The listing builds one solid part. Answer for the finished solid, in the listing's coordinates (mm). Face numbers are marked on the shaded views. A direction names the side the tool comes from. Round coordinates to 2 decimals unless told otherwise and drop trailing zeros. Write each loop counter-clockwise with the first axis right and the second up, starting at its lowest first coordinate (ties: lowest second). Pieces come first, ordered by that corner, then holes.
(1) The mould has two halves that part along X. Classify the marked faces 1, 2 and 3: +X half, -X half, draft (parallel to the pull), parting line (faces both ways), or undercut.
(2) Find the intervals of material crossed by probe 1 along Y at (x, z) = (0, 11); probe 2 along Y at (x, z) = (56.5, -10.5); probe 3 along X at (y, z) = (8, -27), in increasing order.
(3) A cutting plane is placed at A-A, the plane z = -18.5. Give the vertices of the cut face in (x, y).
(4) Each of these flat-tipped pins is pushed along its axis until it touches: pin 1 Ø1.5 at (x, z) = (6, -21.5) entering from -Y; pin 2 Ø8 at (x, z) = (62.5, 24.5) entering from -Y; pin 3 Ø1 at (x, z) = (20.5, 19.5) entering from +Y. Where does it stop, or does it pass through?
(5) A cutting plane is placed at C-C, the plane x = 7. Give the vertices of the cut face in (y, z).
(6) A cutting plane is placed at B-B, the plane y = 0. Give the vertices of the cut face in (x, z), and give its area (4 significant figures).
(7) For the marked faces 4, 5 and 6, determine the directions among +Z, -Z, +X, -X, +Y, -Y from which every point of the face is accessible in a straight line to the end or side of a thin tool.
(8) A cutting plane is placed at D-D, the plane y = 23.5. Give the vertices of the cut face in (x, z).
from build123d import *

# Parameters (mm, degrees)
SKETCH1_R           = 19
BOSS_EXTRUDE1_DEPTH = 32.5
BOSS_EXTRUDE2_START = -9.5
SKETCH2_R           = 5
BOSS_EXTRUDE2_DEPTH = 16
CUT_EXTRUDE2_START  = -16
SKETCH4_R           = 5
CUT_EXTRUDE2_DEPTH  = 16


with BuildPart() as part:
    # Sketch1 → Boss-Extrude1 (new, symmetric)
    with BuildSketch(Plane.XY):
        with BuildLine():
            Line((37.433273968, 19), (50, 19))
            Line((50, 19), (50, 28.5))
            Line((50, 28.5), (0, 28.5))
            ThreePointArc((0, 28.5), (-17.640484356, -22.38444352), (27.710345665, 6.662337662))
            ThreePointArc((27.710345665, 6.662337662), (29.57908326, 15.189643634), (37.433273968, 19))
        make_face()
        Circle(SKETCH1_R, mode=Mode.SUBTRACT)
    extrude(amount=BOSS_EXTRUDE1_DEPTH, both=True)

    # Sketch2 → Boss-Extrude2 (add)
    with BuildSketch(Plane(origin=(0, 28.5, 0), x_dir=(1, 0, 0), z_dir=(0, 1, 0)).offset(BOSS_EXTRUDE2_START)):
        with BuildLine():
            Line((37.5, 20), (37.5, -20))
            ThreePointArc((37.5, -20), (43.725914773, -30.811376164), (56.201736729, -30.853039277))
            Line((56.201736729, -30.853039277), (91.201736729, -10.853039277))
            ThreePointArc((91.201736729, -10.853039277), (97.5, 0), (91.201736729, 10.853039277))
            Line((91.201736729, 10.853039277), (56.201736729, 30.853039277))
            ThreePointArc((56.201736729, 30.853039277), (43.725914773, 30.811376164), (37.5, 20))
        make_face()
        with Locations(Location((50, 20, 0), (0, 0, 270))):
            Circle(SKETCH2_R, mode=Mode.SUBTRACT)
        with Locations(Location((50, -20, 0), (0, 0, 270))):
            Circle(SKETCH2_R, mode=Mode.SUBTRACT)
        with Locations(Location((85, 0, 0), (0, 0, 270))):
            Circle(SKETCH2_R, mode=Mode.SUBTRACT)
    extrude(amount=BOSS_EXTRUDE2_DEPTH)

    # Sketch4 → Cut-Extrude2 (cut)
    with BuildSketch(Plane(origin=(0, 35, 0), x_dir=(1, 0, 0), z_dir=(0, 1, 0)).offset(CUT_EXTRUDE2_START)):
        with Locations(Location((50, -20, 0), (0, 0, 270))):
            Circle(SKETCH4_R)
        with Locations(Location((85, 0, 0), (0, 0, 270))):
            Circle(SKETCH4_R)
        with Locations(Location((50, 20, 0), (0, 0, 270))):
            Circle(SKETCH4_R)
    extrude(amount=CUT_EXTRUDE2_DEPTH, mode=Mode.SUBTRACT)


solid = part.part
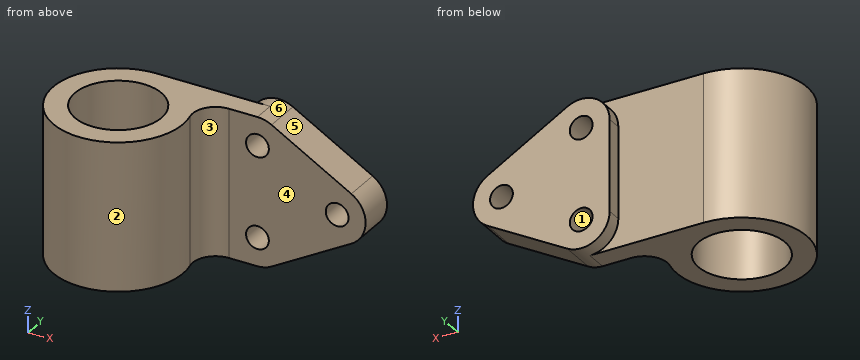
Solutions:
1. face 1: undercut
1. face 2: parting line
1. face 3: +X half
2. probe 1: y = -28.5 to -19, 19 to 28.5
2. probe 2: y = 19 to 35
2. probe 3: x = -27.35 to -17.23, 17.23 to 27.48
3. outline: (0, 28.5) arc R28.5 ccw (long way) to (27.71, 6.66) arc R10 cw to (37.43, 19) - (45.23, 19) - (45.23, 35) - (37.5, 35) - (37.5, 28.5) - close; (54.77, 19) - (77.82, 19) - (77.82, 35) - (54.77, 35) - close; hole circle Ø38 at (0, 0)
4. pin 1: stops at y = -28.01
4. pin 2: stops at y = 19
4. pin 3: stops at y = 28.5
5. outline: (-27.63, -32.5) - (-17.66, -32.5) - (-17.66, 32.5) - (-27.63, 32.5) - close; (17.66, -32.5) - (28.5, -32.5) - (28.5, 32.5) - (17.66, 32.5) - close
6. outline: (-28.5, -32.5) - (-19, -32.5) - (-19, 32.5) - (-28.5, 32.5) - close; (19, -32.5) - (28.5, -32.5) - (28.5, 32.5) - (19, 32.5) - close
6. area: 1,235 mm2
7. face 4: +Z, -Z, +X, -Y
7. face 5: +Z, +X, +Y, -Y
7. face 6: +Z, +Y
8. outline: (-16.12, -32.5) - (50, -32.5) arc R12.5 ccw to (56.2, -30.85) - (91.2, -10.85) arc R12.5 ccw to (91.2, 10.85) - (56.2, 30.85) arc R12.5 ccw to (50, 32.5) - (-16.12, 32.5) - close; hole circle Ø10 at (50, -20); hole circle Ø10 at (50, 20); hole circle Ø10 at (85, 0)
